Answer from the drawing. Dimensions are ordinates in mm from the lowest x, y and z of the part. A direction names the side the tool comes from. Round coordinates to 2 decimals unless told otherwise and drop trailing zeros. Loops run counter-clockwise (first coordinate to the right, second up) from the corner with the lowest first, then second, coordinate; pieces in that order, holes last.
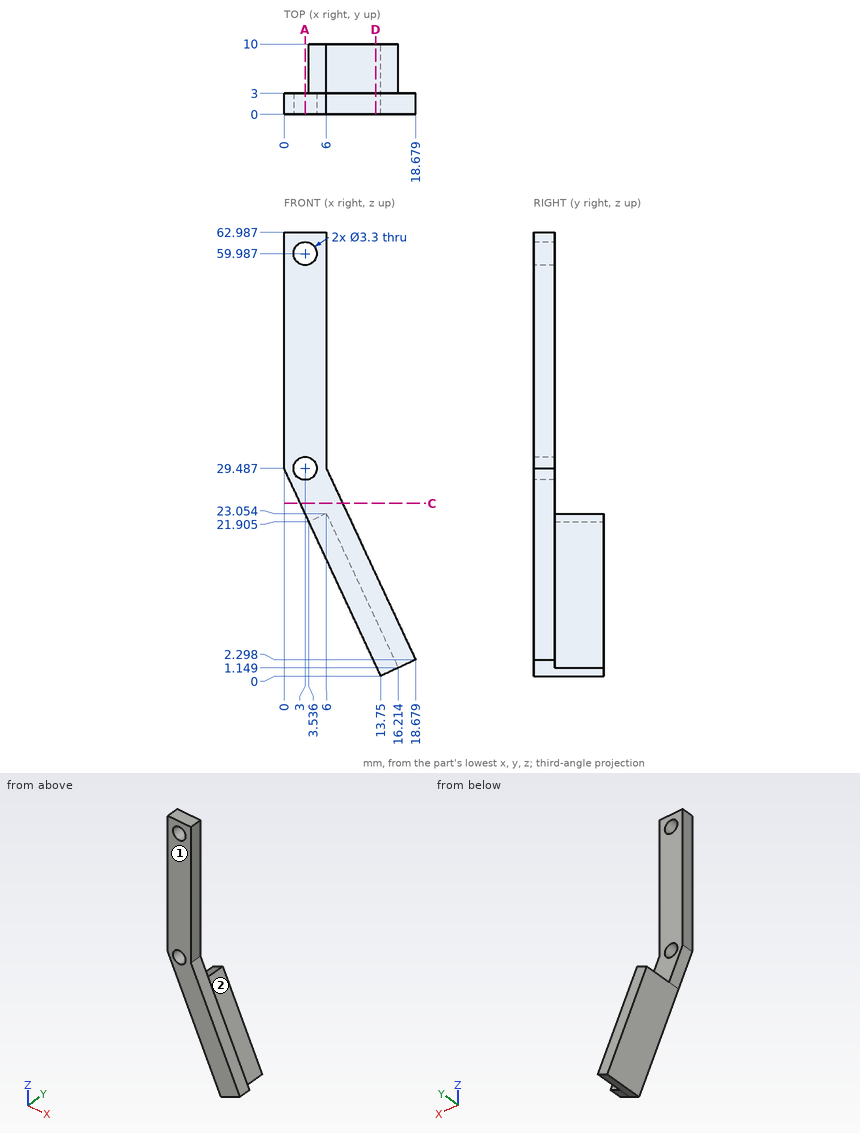
1. Consider probe 1 along X at (y, z) = (2.5, 37); probe 2 along Y at (x, z) = (5.75, 46.5); probe 3 along Z at (x, y) = (13, 3.5) (1 decimal). Determine where each line is inside the solid, lowest interval first.
Answer key:
probe 1: x = 0 to 6
probe 2: y = 0 to 3
probe 3: z = 1.6 to 8
2. Find section C-C (z = 24.5). Write down the section's boundary in (x, y) (1 decimal), then the cut area to 3 significant figures.
Answer key:
outline: (2.3, 0) - (8.3, 0) - (8.3, 3) - (2.3, 3) - close
area: 18.0 mm2
3. Given pin 1 (2.5 mm diameter, centred on y = 2, z = 43, fed in from +X); pin 2 (1.5 mm diameter, centred on x = 16, y = 8.5, fed in from +Z) (1 decimal); pin 3 (3 mm diameter, centred on x = 7, y = 8.5, fed in from -Z), each flat-ended and moving along its own axis, determine where each tip first touches the part or whether it passes through.
Answer key:
pin 1: stops at x = 6
pin 2: stops at z = 3.2
pin 3: stops at z = 11.26
4. Which of the six approach directions +Z, -Z, +X, -X, +Y, -Y give full straight-line access (tool end or side, diameter ignored) to the marked faces 1 and 2?
Answer key:
face 1: +Z, -Z, +X, -X, -Y
face 2: +Z, +X, +Y
5. Find section D-D (x = 13). Write down the section's boundary in (y, z) (1 decimal).
Answer key:
outline: (0, 1.6) - (10, 1.6) - (10, 8) - (3, 8) - (3, 14.5) - (0, 14.5) - close
6. Find section A-A (x = 3). Write down the section's boundary in (y, z).
Answer key:
outline: (0, 23.05) - (3, 23.05) - (3, 27.84) - (0, 27.84) - close; (0, 31.14) - (3, 31.14) - (3, 58.34) - (0, 58.34) - close; (0, 61.64) - (3, 61.64) - (3, 62.99) - (0, 62.99) - close
